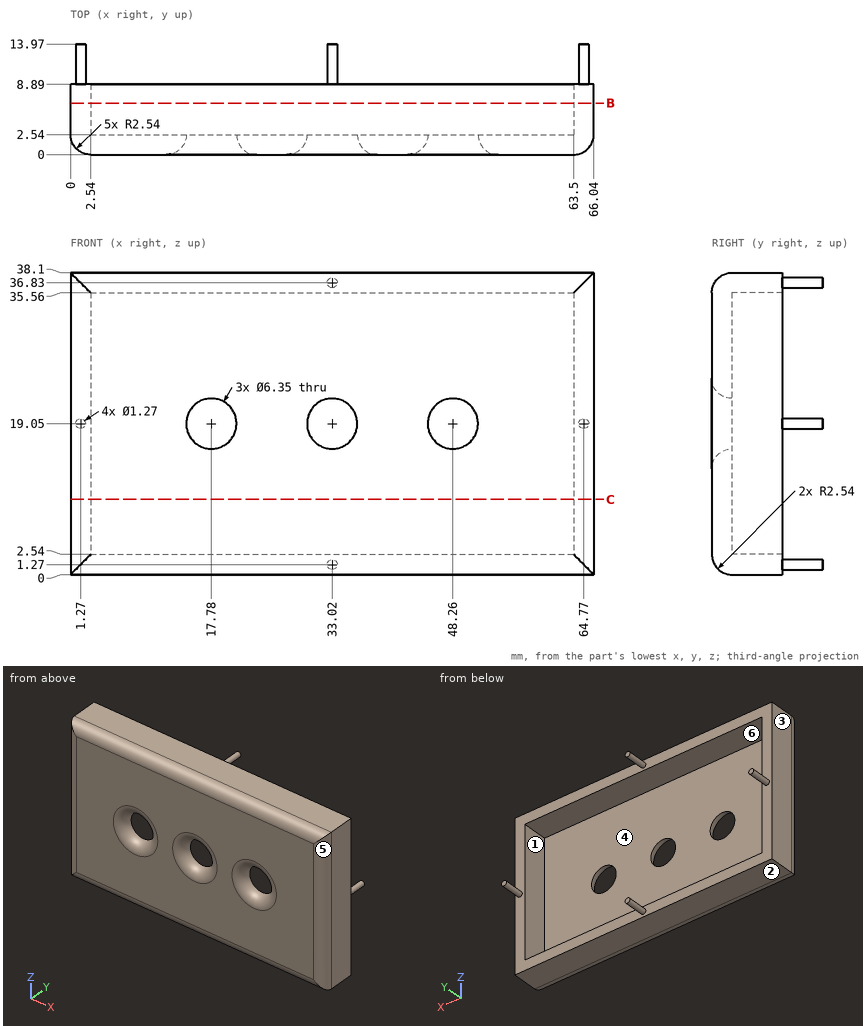
Input: dimensioned drawing with shaded views. Units: mm. Origin: part minimum x, y, z. A direction names the side the tool comes from. Round coordinates to 2 decimals unless told otherwise and drop trailing zeros. Loops run counter-clockwise (first coordinate to the right, second up) from the corner with the lowest first, then second, coordinate; pieces in that order, holes last. Notation, with made-up numbers: M -15.5,88.25 L 16.5,88.25 A17 ccw 16.5,118.25 Z; hole C 68,25.25 d10. An arc over 180 degrees is marked long. Answer in a Markdown table with one row per item. Add a question column.
1. Section C-C (z = 9.5). Output: boundary loops of the cut face in (x, y).
2. Contact query for flat-ended pins moving along their axis: pin 1 (4 mm diameter, centred on x = 17.78, z = 19.05, fed in from +Y); pin 2 (2 mm diameter, centred on x = 37.5, z = 7.5, fed in from +Y); pin 3 (19 mm diameter, centred on x = 25.5, z = 9.5, fed in from +Y); pin 4 (1 mm diameter, centred on y = 10.5, z = 19, fed in from +X) (3 decimals). Output: stop coordinate, or through.
3. Ray query, probe 1 along X at (y, z) = (2.5, 19.05); probe 2 along X at (y, z) = (7.5, 35); probe 3 along Z at (x, y) = (33.02, 2.5). Return the intervals inside material, ascending.
4. Set-up query: the marked faces 5 and 6. Return all of +Z, -Z, +X, -X, +Y, -Y with unobstructed straight access to the full face (end or side cutting, diameter ignored); none if empty.
5. Mould query, pull axis X, two halves, no side actions, for the marked faces 1, 2, 3 and 4. Classes: released by +X, released by -X, zero draft, split by the parting line, or undercut.
6. Section B-B (y = 6.5). Output: boundary loops of the cut face in (x, z).
Values follow:
| question | item | result |
|---|---|---|
| 1 | outline | M 0,2.54 A2.54 ccw 2.54,0 L 63.5,0 A2.54 ccw 66.04,2.54 L 66.04,8.89 L 63.5,8.89 L 63.5,2.54 L 2.54,2.54 L 2.54,8.89 L 0,8.89 Z |
| 2 | pin 1 | through |
| 2 | pin 2 | y = 2.54 |
| 2 | pin 3 | y = 8.89 |
| 2 | pin 4 | x = 65.405 |
| 3 | probe 1 | 0 to 14.6, 20.96 to 29.84, 36.2 to 45.08, 51.44 to 66.04 |
| 3 | probe 2 | 0 to 2.54, 63.5 to 66.04 |
| 3 | probe 3 | 0 to 15.87, 22.23 to 38.1 |
| 4 | face 5 | +Z, -Z, +X, -Y |
| 4 | face 6 | +Y |
| 5 | face 1 | undercut |
| 5 | face 2 | zero draft |
| 5 | face 3 | released by -X |
| 5 | face 4 | undercut |
| 6 | outline | M 0,0 L 66.04,0 L 66.04,38.1 L 0,38.1 Z; hole M 2.54,2.54 L 63.5,2.54 L 63.5,35.56 L 2.54,35.56 Z |
